from build123d import *

# Parameters (mm, degrees)
F0_R          = 5
F1_DEPTH      = 25
F2_R          = 4.8
F3_DEPTH      = 3
F5_DEPTH      = 5
F5_DEPTH_BACK = 23
F6_W          = 40
F6_H          = 20
F6_R          = 1.5
F7_DEPTH      = 10
F9_DEPTH      = 10
F10_T1_DEPTH  = 34.9696394511
F10_T3_DEPTH  = 35
F10_T5_DEPTH  = 34.9715357564
F11_R         = 0.5
F12_R         = 6
F13_DEPTH     = 4.9
F14_R         = 2.5
F15_DEPTH     = 65


# Not quite as in the source:
# - a fillet or chamfer that OpenCascade refuses, or shapes differently, is made with other operations: its cross-section is extruded or revolved along the edge and cut away or added
# - a feature names something its author has since deleted; it is built from what else it names


with BuildPart() as f1:
    # F0 (on Right) → F1 (new body)
    with BuildSketch(Plane.YZ):
        Circle(F0_R)
    extrude(amount=-F1_DEPTH)

    # F2 (on face) → F3 (join)
    with BuildSketch(Plane.YZ):
        Circle(F2_R)
    extrude(amount=F3_DEPTH)

    # F4 (on face) → F5 (join, two sides)
    with BuildSketch(Plane.YZ.offset(3)) as f5_sk:
        Polygon((-4.5650712782, -1.483281573), (0, -4.8), (4.5650712782, -1.483281573), (2.821369211, 3.883281573), (-2.821369211, 3.883281573), align=None)
    extrude(amount=F5_DEPTH)
    extrude(f5_sk.sketch, amount=-F5_DEPTH_BACK)

    # F6 (on face) → F7 (join)
    with BuildSketch(Plane(origin=(-25, 0, 0), x_dir=(0, -1, 0), z_dir=(-1, 0, 0))):
        Rectangle(F6_W, F6_H)
        with Locations((-15, 0)):
            Circle(F6_R, mode=Mode.SUBTRACT)
        with BuildLine():
            ThreePointArc((13.5, 0), (15, 1.5), (16.5, 0))
            ThreePointArc((16.5, 0), (15, -1.5), (13.5, 0))
        make_face(mode=Mode.SUBTRACT)
    extrude(amount=-F7_DEPTH)

    # F8 (on face) → F9 (cut)
    with BuildSketch(Plane(origin=(-25, 0, 0), x_dir=(0, -1, 0), z_dir=(-1, 0, 0))):
        with BuildLine():
            Line((15.0452693954, 10), (14.9885289893, 10))
            Line((14.9885289893, 10), (14.7385289893, 10))
            Line((14.7385289893, 10), (14.8751285557, 6.9943249556))
            ThreePointArc((14.8751285557, 6.9943249556), (15.0159151334, 6.8760173486), (15.1222554927, 7.0260482732))
            Line((15.1222554927, 7.0260482732), (15.2385289893, 10))
            Line((15.2385289893, 10), (15.0452693954, 10))
        make_face()
        with BuildLine():
            Line((-14.9398591969, 10.0056750444), (-14.9965996031, 10.0056750444))
            Line((-14.9965996031, 10.0056750444), (-15.2465996031, 10.0056750444))
            Line((-15.2465996031, 10.0056750444), (-15.1100000367, 7))
            ThreePointArc((-15.1100000367, 7), (-14.9692134589, 6.881692393), (-14.8628730997, 7.0317233176))
            Line((-14.8628730997, 7.0317233176), (-14.7465996031, 10.0056750444))
            Line((-14.7465996031, 10.0056750444), (-14.9398591969, 10.0056750444))
        make_face()
    extrude(amount=-F9_DEPTH, mode=Mode.SUBTRACT)

    # F10: fillet of radius 5 on 4 edges, made by hand

    # F10_s2 → F10_t1 (cut)
    with BuildSketch(Plane.YZ.offset(-37.4848197255)):
        with BuildLine():
            ThreePointArc((20, 5.0060721098), (18.6215817291, 8.4534110516), (15.2463416881, 10))
            Line((15.2463416881, 10), (20, 10))
            Line((20, 10), (20, 5.0060721098))
        make_face()
    extrude(amount=F10_T1_DEPTH, mode=Mode.SUBTRACT)

    # F10_s4 → F10_t3 (cut)
    with BuildSketch(Plane.YZ.offset(-37.5)):
        with BuildLine():
            ThreePointArc((15, -10), (18.5355339059, -8.5355339059), (20, -5))
            Line((20, -5), (20, -10))
            Line((20, -10), (15, -10))
        make_face()
        with BuildLine():
            ThreePointArc((-20, -5), (-18.5355339059, -8.5355339059), (-15, -10))
            Line((-15, -10), (-20, -10))
            Line((-20, -10), (-20, -5))
        make_face()
    extrude(amount=F10_T3_DEPTH, mode=Mode.SUBTRACT)

    # F10_s6 → F10_t5 (cut)
    with BuildSketch(Plane.YZ.offset(-37.4857678782)):
        with BuildLine():
            ThreePointArc((-20, 5.0056928487), (-18.6188841475, 8.4558635006), (-15.2385289893, 10))
            Line((-15.2385289893, 10), (-20, 10))
            Line((-20, 10), (-20, 5.0056928487))
        make_face()
    extrude(amount=F10_T5_DEPTH, mode=Mode.SUBTRACT)

    # F11
    f11_edges = [f1.edges().sort_by_distance(p)[0] for p in [
        (-20, -14.738529, 10),
        (-20, 14.746821, 10),
        (-20, 15.246342, 10),
        (-20, -15.238529, 10),
    ]]
    fillet(f11_edges, radius=F11_R)

    # F12 (on face) → F13 (join)
    with BuildSketch(Plane.YZ.offset(-15)):
        Circle(F12_R)
    extrude(amount=F13_DEPTH)

    # F14 (on face) → F15 (cut)
    with BuildSketch(Plane.YZ.offset(8)):
        Circle(F14_R)
    extrude(amount=-F15_DEPTH, mode=Mode.SUBTRACT)


solid = f1.part
The model under review builds one solid part; all positions refer to its coordinate system, in mm. A direction names the side the tool comes from. Give positions to 0.01 mm unless a question says otherwise; leave off trailing zeros. Loops run counter-clockwise (first coordinate to the right, second up) from the corner with the lowest first, then second, coordinate; pieces in that order, holes last. Notation, with made-up numbers: (80.5, 1) -> (108.5, 1) arc R12 cw to (108.5, 13) -> close; hole circle Ø7 at (-5.5, -39). An arc over 180 degrees is marked (long way). Write each question's results on one line, items separated by ' | '.
1) Take a section at A-A, the plane x = -20. Give the boundary of the cut face in (y, z) (3 decimals).
Conclusion:
outline: (-20, -5) arc R5 ccw to (-15, -10) -> (15, -10) arc R5 ccw to (20, -5) -> (20, 5.006) arc R5 ccw to (15.802, 9.941) arc R0.5 ccw to (15.222, 9.471) -> (15.11, 7) arc R0.125 cw (long way) to (14.863, 7.032) -> (14.766, 9.52) arc R0.5 ccw to (14.266, 10) -> (-14.261, 10) arc R0.5 ccw to (-14.76, 9.523) -> (-14.875, 6.994) arc R0.125 cw (long way) to (-15.122, 7.026) -> (-15.218, 9.468) arc R0.5 ccw to (-15.797, 9.942) arc R5 ccw to (-20, 5.006) -> close; hole circle Ø3 at (-15, 0); hole circle Ø5 at (0, 0); hole circle Ø3 at (15, 0)
2) Take a section at B-B, the plane x = 4.5. Give the boundary of the cut face in (y, z), plus the area to 3 significant figures.
Conclusion:
outline: (-4.57, -1.48) -> (0, -4.8) -> (4.57, -1.48) -> (2.82, 3.88) -> (-2.82, 3.88) -> close; hole circle Ø5 at (0, 0) | area: 35.1 mm^2
3) Take a section at C-C, the plane z = 0. Count the separate pieces of the cut face and the enclosed holes in it, plus the area to 3 significant figures.
Conclusion:
separate pieces: 4 | enclosed holes: 0 | area: 404 mm^2
4) For line 1 along Z through (x, y) = (-19, -15) (3 decimals); line 2 along X through (y, z) = (-7.5, 2); line 3 along Y through (x, z) = (-0.5, 1), list the stretches that pass through material, from the lowest coordinate up. Write a range as from..to.
Conclusion:
line 1: z = -10..-1.5, 1.5..6.875 | line 2: x = -25..-15 | line 3: y = -4.9..-2.29, 2.29..4.9
5) Take a section at D-D, the plane z = 8.5. Give the boundary of the cut face in (x, y), plus the area to 3 significant figures.
Conclusion:
outline: (-25, -18.58) -> (-15, -18.58) -> (-15, -15.18) -> (-25, -15.18) -> close; (-25, -14.81) -> (-15, -14.81) -> (-15, 14.81) -> (-25, 14.81) -> close; (-25, 15.18) -> (-15, 15.18) -> (-15, 18.58) -> (-25, 18.58) -> close | area: 364 mm^2
6) Tool access review of faces 1 (the face through (1.48, 2.58, 4.05)), 2 (the face through (5.465, 3.705, 1.162)), 3 (the face through (3, 2.6, -3.5)), 4 (the face through (5, 0, 3.883)), 5 (the face through (-20.07, 14.815, 8.258)): name each direction out of +Z, -Z, +X, -X, +Y, -Y from which nothing blocks a thin tool from reaching the whole face with its end or side.
Conclusion:
face 1: +X | face 2: +Z, +X, +Y | face 3: -Z, +X, +Y | face 4: +Z, +X, +Y, -Y | face 5: +Z, +X, -X
7) Insertion check: pin 1 Ø1.5 at (x, z) = (-4, 0.5) entering from +Y; pin 2 Ø6 at (y, z) = (6.5, 3.5) entering from +X; pin 3 Ø6 at (x, y) = (-11, 3.5) entering from -Z; pin 4 Ø2.5 at (y, z) = (15, 0) entering from -X. Each pin has a flat end and moves straight along its axis. Give the tip position at first contact, or say it passes through.
Conclusion:
pin 1: stops at y = 5 | pin 2: stops at x = 3 | pin 3: stops at z = -5.98 | pin 4: passes through
